```python
from build123d import *

# Parameters (mm, degrees)
SKETCH2_R               = 3.175
BOSS_EXTRUDE1_DEPTH     = 25.4
CUT_EXTRUDE1_DEPTH      = 39.1
CUT_EXTRUDE1_DEPTH_BACK = 39.1
SKETCH3_R               = 3.175
SKETCH4_R               = 4.7625
CUT_EXTRUDE2_DEPTH      = 22.225


with BuildPart() as part:
    # Sketch2 → Boss-Extrude1 (new body)
    with BuildSketch(Plane(origin=(0, 0, 0), x_dir=(1, 0, 0), z_dir=(0, 1, 0))):
        with BuildLine():
            Line((12.7, 12.7), (12.7, -12.7))
            ThreePointArc((12.7, -12.7), (0, -25.4), (-12.7, -12.7))
            Line((-12.7, -12.7), (-12.7, 12.7))
            ThreePointArc((-12.7, 12.7), (0, 25.4), (12.7, 12.7))
        make_face()
        with Locations(Location((0, 12.7, 0), (0, 0, 270))):
            Circle(SKETCH2_R, mode=Mode.SUBTRACT)
        with Locations(Location((0, -12.7, 0), (0, 0, 270))):
            Circle(SKETCH2_R, mode=Mode.SUBTRACT)
    extrude(amount=BOSS_EXTRUDE1_DEPTH)

    # Sketch3 → Cut-Extrude1 (cut, two sides: drawn at the far end of the back side and taken through both)
    with BuildSketch(Plane(origin=(0, 0, 0), x_dir=(0, 0, -1), z_dir=(1, 0, 0)).offset(-CUT_EXTRUDE1_DEPTH_BACK)):
        with Locations((0, 11.1125)):
            Circle(SKETCH3_R)
        with BuildLine():
            Line((-25.4, 7.90575), (-19.186582283, 7.90575))
            ThreePointArc((-19.186582283, 7.90575), (-11.300258027, 9.761112271), (-5.068357629, 14.937973951))
            ThreePointArc((-5.068357629, 14.937973951), (0, 17.4625), (5.068357629, 14.937973951))
            ThreePointArc((5.068357629, 14.937973951), (11.300258027, 9.761112271), (19.186582283, 7.90575))
            Line((19.186582283, 7.90575), (25.4, 7.90575))
            Line((25.4, 7.90575), (25.4, 30.015599029))
            Line((25.4, 30.015599029), (-31.207208801, 35.201112742))
            Line((-31.207208801, 35.201112742), (-25.4, 7.90575))
        make_face()
    extrude(amount=CUT_EXTRUDE1_DEPTH + CUT_EXTRUDE1_DEPTH_BACK, mode=Mode.SUBTRACT)

    # Sketch4 → Cut-Extrude2 (cut)
    with BuildSketch(Plane(origin=(0, 25.4, 0), x_dir=(1, 0, 0), z_dir=(0, 1, 0))):
        with Locations(Location((0, -12.7, 0), (0, 0, 270))):
            Circle(SKETCH4_R)
        with Locations(Location((0, 12.7, 0), (0, 0, 270))):
            Circle(SKETCH4_R)
    extrude(amount=-CUT_EXTRUDE2_DEPTH, mode=Mode.SUBTRACT)


solid = part.part
```
Input: part model. Units: mm. Frame: model coordinates. A direction names the side the tool comes from. Coordinates: 2 decimals unless noted, no trailing zeros. Write each loop counter-clockwise with the first axis right and the second up, starting at its lowest first coordinate (ties: lowest second). Pieces come first, ordered by that corner, then holes. Notation, with made-up numbers: (49, 56.25) -> (91, 56.25) arc R17 cw to (91, 71.25) -> close; hole circle Ø1 at (-25.5, -28). An arc over 180 degrees is marked (long way). Answer as a JSON object with one key per item and string values.
1. Section A-A on z = 0. Return the cut outline in (x, y).
Result set:
{"outline": "(-12.7, 0) -> (12.7, 0) -> (12.7, 7.94) -> (-12.7, 7.94) -> close; (-12.7, 14.29) -> (12.7, 14.29) -> (12.7, 17.46) -> (-12.7, 17.46) -> close"}
2. Mould query, pull axis X, two halves, no side actions, for faces 1 (the face through (-1, 3.175, 16)), 2 (the face through (-0.18, 17.46, 0.08)), 3 (the face through (0.279, 3.49, 25.397)). Classes: released by +X, released by -X, zero draft, split by the parting line, or undercut.
Result set:
{"face 1": "undercut", "face 2": "zero draft", "face 3": "split by the parting line"}
3. First-contact query: P1, Ø3, axis at x = 0.5, z = -21.5, coming from the +Y side; P2, Ø5, axis at x = 0.5, z = -14.5, coming from the +Y side (3 decimals); P3, Ø7.5, axis at x = -2, z = 15, coming from the +Y side. Flat tips, straight axial feed; report the tip coordinate or a pass-through.
Result set:
{"P1": "stops at y = 7.91", "P2": "stops at y = 3.175", "P3": "stops at y = 9.24"}
4. Section C-C on x = -2.5. Count the separate pieces of the cut face and the enclosed holes in it, then the cut area to 3 significant figures.
Result set:
{"separate pieces": "3", "enclosed holes": "1", "area": "390 mm2"}
5. Section B-B on y = 1. Return the cut outline in (x, z) (3 decimals), then the cut area to 3 significant figures.
Result set:
{"outline": "(-12.7, -12.7) arc R12.7 ccw to (12.7, -12.7) -> (12.7, 12.7) arc R12.7 ccw to (-12.7, 12.7) -> close; hole circle Ø6.35 at (0, -12.7); hole circle Ø6.35 at (0, 12.7)", "area": "1,090 mm2"}
6. Material intervals for line 1 (Z direction, x = 0, y = 7.25); line 2 (X direction, y = 2.3, z = -12.7) (3 decimals); line 3 (Z direction, x = 0, y = 2) (3 decimals), sorted ascending. Write a range as from..to.
Result set:
{"line 1": "z = -25.4..-17.46, -7.94..7.94, 17.46..25.4", "line 2": "x = -12.7..-3.175, 3.175..12.7", "line 3": "z = -25.4..-15.875, -9.525..9.525, 15.875..25.4"}
7. Access query for faces 4 (the face through (0, 7.906, -22)), 5 (the face through (0.209, 6.646, 7.942)), 6 (the face through (12.7, 7, 0)), 7 (the face through (0, 7.906, 22)), 8 (the face through (-0.178, 8.013, 0.688)). Directions: +Z, -Z, +X, -X, +Y, -Y. A direction counts if a zero-diameter tool reaches every point of the face in a straight line with its end or side. Return the directions, or none.
Result set:
{"face 4": "-Z, +X, -X, +Y", "face 5": "+Y", "face 6": "+Z, -Z, +X, +Y, -Y", "face 7": "+Z, +X, -X, +Y", "face 8": "+X, -X"}
